CAD build for the part. Positions are in the model's coordinates, mm. A direction names the side the tool comes from. Coordinates: 2 decimals unless noted, no trailing zeros. Order: outer loops, then holes, each group sorted by start corner. A loop starts at its lowest first (then second) coordinate and runs counter-clockwise, first axis right, second up. Notation, with made-up numbers: (83, 16) - (136, 16) arc R18 cw to (136, 23) - close; hole circle Ø6 at (47.25, -35.5). An arc over 180 degrees is marked (long way). Write each question's results on one line, items separated by ' | '. Start each with the question number.
Q1. Band-saw the part on A-A, the plane x = 38.1. Write the cut outline in (y, z), then the cut area to 3 significant figures.
Q2. Band-saw the part on B-B, the plane x = 22. Write the cut outline in (y, z), then the cut area to 3 significant figures.
Q3. Band-saw the part on C-C, the plane x = 47. Write the cut outline in (y, z).
Q4. Wall check: probe 1 along Y at (x, z) = (12.7, 0.85); probe 2 along Z at (x, y) = (30, 9.25); probe 3 along Y at (x, z) = (31, 2.2). Give the ranges that are in metal, low to high.
Q5. Which spindle directions (+Z, -Z, +X, -X, +Y, -Y) get a long thin tool onto all of the face, cutting with end or side? Do faces 5 (the flat face through (9.9, 8, 2)), 6 (the flat face through (47, 2, 2.6)), 7 (the flat face through (31.39, 8, 2)), 8 (the flat face through (47, 9.05, 2)). Say none if no direction does.
Q6. Pull direction X, two halves, no side cores. Call faces 1 (the flat face through (16, 4, 2.4)), 2 (the flat face through (0.9, 8, 2)), 3 (the flat face through (8, 7.55, 2)), 4 (the flat face through (29, 4, 2.4)): released by +X, released by -X, zero draft, split by the parting line, or undercut.
Q7. Pin check, flat tips, straight feed: P1, Ø3, axis at x = 22.225, y = 3.81, coming from the +Z side; P2, Ø0.5, axis at x = 9, z = 2, coming from the -Y side; P3, Ø0.8, axis at y = 8, z = 2.5, coming from the +X side. Stop position of each tip, or through.
Autodesk Fusion 360 part; units mm, degrees
sketch "Sketch1" plane through (0, 0, 0) normal (0, 0, 1) x (1, 0, 0)
  line L0 (0, 0) -> (50.8, 0)
  line L1 (50.8, 0) -> (50.8, 10.16)
  line L2 (50.8, 10.16) -> (0, 10.16)
  line L3 (0, 10.16) -> (0, 0)
  line L4 (25.4, 10.16) -> (25.4, 0) construction
  circle A0 centre (12.7, 8.128) radius 1.1
  circle A1 centre (38.1, 8.128) radius 1.1
  dimension "d1" = 50.8
  dimension "d2" = 10.16
  dimension "d3" = 2.2
  dimension "d4" = 2.2
  dimension "d5" = 12.7
  dimension "d6" = 38.1
  dimension "d7" = 8.128
  dimension "d8" = 8.128
extrude "Extrude1" add sketch "Sketch1" along normal blind 1.6
sketch "Sketch2" plane through (0, 0, 1.6) normal (0, 0, 1) x (-1, 0, 0)
  circle A0 centre (-12.7, -8.128) radius 1.1
  circle A1 centre (-38.1, -8.128) radius 1.1
  line L0 (0, -10.16) -> (0, 0)
  line L1 (0, 0) -> (-50.8, 0)
  line L2 (-50.8, 0) -> (-50.8, -10.16)
  line L3 (-50.8, -10.16) -> (0, -10.16)
  line L4 (-5.675, -1.31) -> (-0.675, -1.31)
  line L5 (-0.675, -1.31) -> (-0.675, -6.31)
  line L6 (-0.675, -6.31) -> (-5.675, -6.31)
  line L7 (-5.675, -6.31) -> (-5.675, -1.31)
  line L8 (-5.675, -1.31) -> (-0.675, -6.31) construction
  line L9 (-0.675, -1.31) -> (-5.675, -6.31) construction
  circle A2 centre (-3.175, -3.81) radius 1.75
  line L10 (-7.025, -1.31) -> (-7.025, -6.31)
  line L11 (-7.025, -6.31) -> (-12.025, -6.31)
  line L12 (-12.025, -1.31) -> (-7.025, -1.31)
  line L13 (-12.025, -6.31) -> (-12.025, -1.31)
  circle A3 centre (-9.525, -3.81) radius 1.75
  line L14 (-13.375, -1.31) -> (-13.375, -6.31)
  line L15 (-13.375, -6.31) -> (-18.375, -6.31)
  line L16 (-18.375, -1.31) -> (-13.375, -1.31)
  line L17 (-18.375, -6.31) -> (-18.375, -1.31)
  circle A4 centre (-15.875, -3.81) radius 1.75
  line L18 (-19.725, -1.31) -> (-19.725, -6.31)
  line L19 (-19.725, -6.31) -> (-24.725, -6.31)
  line L20 (-24.725, -1.31) -> (-19.725, -1.31)
  line L21 (-24.725, -6.31) -> (-24.725, -1.31)
  circle A5 centre (-22.225, -3.81) radius 1.75
  line L22 (-26.075, -1.31) -> (-26.075, -6.31)
  line L23 (-26.075, -6.31) -> (-31.075, -6.31)
  line L24 (-31.075, -1.31) -> (-26.075, -1.31)
  line L25 (-31.075, -6.31) -> (-31.075, -1.31)
  circle A6 centre (-28.575, -3.81) radius 1.75
  line L26 (-32.425, -1.31) -> (-32.425, -6.31)
  line L27 (-32.425, -6.31) -> (-37.425, -6.31)
  line L28 (-37.425, -1.31) -> (-32.425, -1.31)
  line L29 (-37.425, -6.31) -> (-37.425, -1.31)
  circle A7 centre (-34.925, -3.81) radius 1.75
  line L30 (-38.775, -1.31) -> (-38.775, -6.31)
  line L31 (-38.775, -6.31) -> (-43.775, -6.31)
  line L32 (-43.775, -1.31) -> (-38.775, -1.31)
  line L33 (-43.775, -6.31) -> (-43.775, -1.31)
  circle A8 centre (-41.275, -3.81) radius 1.75
  line L34 (-45.125, -1.31) -> (-45.125, -6.31)
  line L35 (-45.125, -6.31) -> (-50.125, -6.31)
  line L36 (-50.125, -1.31) -> (-45.125, -1.31)
  line L37 (-50.125, -6.31) -> (-50.125, -1.31)
  circle A9 centre (-47.625, -3.81) radius 1.75
  point P0 (-3.175, -3.81)
  dimension "d13" = 5
  dimension "d14" = 5
  dimension "d15" = 3.175
  dimension "d16" = 3.81
  dimension "d17" = 3.5
  dimension "d20" = -6.35
  dimension "d21" = 0
extrude "Extrude2" add sketch "Sketch2" along normal blind 1 draft 1 contours L4 L5 L6 L7 | A2 | L10 L11 L12 L13 | A3 | L14 L15 L16 L17 | A4 | L18 L19 L20 L21 | A5 | L22 L23 L24 L25 | A6 | L26 L27 L28 L29 | A7 | L30 L31 L32 L33 | A8 | L34 L35 L36 L37 | A9
extrude "Extrude3" cut sketch "Sketch2" against normal blind 0.2 from surface at 1 contours A2 | A3 | A4 | A5 | A6 | A7 | A8 | A9
sketch "Sketch3" plane through (0, 0, 1.6) normal (0, 0, 1) x (-1, 0, 0)
  line L0 (-50.125, -6.31) -> (-50.125, -1.31)
  line L1 (-50.125, -1.31) -> (-45.125, -1.31)
  line L2 (-45.125, -1.31) -> (-45.125, -6.31)
  line L3 (-45.125, -6.31) -> (-50.125, -6.31)
  line L4 (-24.725, -6.31) -> (-24.725, -1.31)
  line L5 (-24.725, -1.31) -> (-19.725, -1.31)
  line L6 (-19.725, -1.31) -> (-19.725, -6.31)
  line L7 (-19.725, -6.31) -> (-24.725, -6.31)
  line L8 (-5.675, -6.31) -> (-5.675, -1.31)
  line L9 (-5.675, -1.31) -> (-0.675, -1.31)
  line L10 (-0.675, -1.31) -> (-0.675, -6.31)
  line L11 (-0.675, -6.31) -> (-5.675, -6.31)
  line L12 (-31.075, -6.31) -> (-31.075, -1.31)
  line L13 (-31.075, -1.31) -> (-26.075, -1.31)
  line L14 (-26.075, -1.31) -> (-26.075, -6.31)
  line L15 (-26.075, -6.31) -> (-31.075, -6.31)
  line L16 (-43.775, -6.31) -> (-43.775, -1.31)
  line L17 (-43.775, -1.31) -> (-38.775, -1.31)
  line L18 (-38.775, -1.31) -> (-38.775, -6.31)
  line L19 (-38.775, -6.31) -> (-43.775, -6.31)
  line L20 (-18.375, -6.31) -> (-18.375, -1.31)
  line L21 (-18.375, -1.31) -> (-13.375, -1.31)
  line L22 (-13.375, -1.31) -> (-13.375, -6.31)
  line L23 (-13.375, -6.31) -> (-18.375, -6.31)
  line L24 (-12.025, -6.31) -> (-12.025, -1.31)
  line L25 (-12.025, -1.31) -> (-7.025, -1.31)
  line L26 (-7.025, -1.31) -> (-7.025, -6.31)
  line L27 (-7.025, -6.31) -> (-12.025, -6.31)
  line L28 (-37.425, -6.31) -> (-37.425, -1.31)
  line L29 (-37.425, -1.31) -> (-32.425, -1.31)
  line L30 (-32.425, -1.31) -> (-32.425, -6.31)
  line L31 (-32.425, -6.31) -> (-37.425, -6.31)
  circle A0 centre (-12.7, -8.128) radius 1.1
  circle A1 centre (-38.1, -8.128) radius 1.1
  line L32 (0, -10.16) -> (0, 0)
  line L33 (0, 0) -> (-50.8, 0)
  line L34 (-50.8, 0) -> (-50.8, -10.16)
  line L35 (-50.8, -10.16) -> (0, -10.16)
  line L36 (-0.9, -9.05) -> (-3.9, -9.05)
  line L37 (-3.9, -9.05) -> (-3.9, -7.55)
  line L38 (-3.9, -7.55) -> (-0.9, -7.55)
  line L39 (-0.9, -7.55) -> (-0.9, -9.05)
  line L40 (-2.4, -9.05) -> (-2.4, -7.55) construction
  line L41 (-3.9, -8.3) -> (-0.9, -8.3) construction
  line L42 (-6.9, -7.55) -> (-6.9, -9.05)
  line L43 (-6.9, -9.05) -> (-9.9, -9.05)
  line L44 (-9.9, -7.55) -> (-6.9, -7.55)
  line L45 (-9.9, -9.05) -> (-9.9, -7.55)
  line L46 (-15.4, -9.05) -> (-18.4, -9.05)
  line L47 (-18.4, -9.05) -> (-18.4, -7.55)
  line L48 (-18.4, -7.55) -> (-15.4, -7.55)
  line L49 (-15.4, -7.55) -> (-15.4, -9.05)
  line L50 (-16.9, -9.05) -> (-16.9, -7.55) construction
  line L51 (-18.4, -8.3) -> (-15.4, -8.3) construction
  line L52 (-23.73, -7.55) -> (-20.73, -7.55)
  line L53 (-20.73, -7.55) -> (-20.73, -9.05)
  line L54 (-20.73, -9.05) -> (-23.73, -9.05)
  line L55 (-23.73, -9.05) -> (-23.73, -7.55)
  line L56 (-29.06, -7.55) -> (-26.06, -7.55)
  line L57 (-26.06, -7.55) -> (-26.06, -9.05)
  line L58 (-26.06, -9.05) -> (-29.06, -9.05)
  line L59 (-29.06, -9.05) -> (-29.06, -7.55)
  line L60 (-34.39, -7.55) -> (-31.39, -7.55)
  line L61 (-31.39, -7.55) -> (-31.39, -9.05)
  line L62 (-31.39, -9.05) -> (-34.39, -9.05)
  line L63 (-34.39, -9.05) -> (-34.39, -7.55)
  line L64 (-39.72, -9.05) -> (-42.72, -9.05)
  line L65 (-42.72, -9.05) -> (-42.72, -7.55)
  line L66 (-42.72, -7.55) -> (-39.72, -7.55)
  line L67 (-39.72, -7.55) -> (-39.72, -9.05)
  line L68 (-41.22, -9.05) -> (-41.22, -7.55) construction
  line L69 (-39.72, -8.3) -> (-42.72, -8.3) construction
  line L70 (-32.89, -9.05) -> (-32.89, -7.55) construction
  line L71 (-45.94, -7.55) -> (-45.94, -9.05)
  line L72 (-45.94, -9.05) -> (-48.94, -9.05)
  line L73 (-48.94, -7.55) -> (-45.94, -7.55)
  line L74 (-48.94, -9.05) -> (-48.94, -7.55)
  dimension "d27" = 3
  dimension "d28" = 1.5
  dimension "d29" = 2.4
  dimension "d30" = 8.3
  dimension "d33" = -6
  dimension "d34" = 0
  dimension "d35" = 3
  dimension "d36" = 1.5
  dimension "d37" = 14.5
  dimension "d40" = -5.33
  dimension "d41" = 0
  dimension "d42" = 3
  dimension "d43" = 1.5
  dimension "d44" = 8.33
  dimension "d47" = -6.22
  dimension "d48" = 0
extrude "Extrude4" add sketch "Sketch3" along normal blind 1 contours L36 L37 L38 L39 | L42 L43 L44 L45 | L46 L47 L48 L49 | L52 L53 L54 L55 | L56 L57 L58 L59 | L60 L61 L62 L63 | L64 L65 L66 L67 | L71 L72 L73 L74
Results below:
1) outline: (0, 0) - (7.03, 0) - (7.03, 1.6) - (0, 1.6) - close; (9.23, 0) - (10.16, 0) - (10.16, 1.6) - (9.23, 1.6) - close | area: 12.7 mm²
2) outline: (0, 0) - (10.16, 0) - (10.16, 1.6) - (9.05, 1.6) - (9.05, 2.6) - (7.55, 2.6) - (7.55, 1.6) - (6.31, 1.6) - (6.33, 2.6) - (5.55, 2.6) - (5.55, 2.4) - (2.07, 2.4) - (2.07, 2.6) - (1.29, 2.6) - (1.31, 1.6) - (0, 1.6) - close | area: 22.1 mm²
3) outline: (0, 0) - (10.16, 0) - (10.16, 1.6) - (9.05, 1.6) - (9.05, 2.6) - (7.55, 2.6) - (7.55, 1.6) - (6.31, 1.6) - (6.33, 2.6) - (5.44, 2.6) - (5.44, 2.4) - (2.18, 2.4) - (2.18, 2.6) - (1.29, 2.6) - (1.31, 1.6) - (0, 1.6) - close
4) probe 1: y = 0 to 7.03, 9.23 to 10.16 | probe 2: z = 0 to 1.6 | probe 3: y = 1.3 to 6.32
5) face 5: +Z, +Y | face 6: +Z, +X, -X, +Y, -Y | face 7: +Z, +Y, -Y | face 8: +Z, +X, -X, +Y
6) face 1: undercut | face 2: released by -X | face 3: zero draft | face 4: undercut
7) P1: stops at z = 2.4 | P2: stops at y = 1.3 | P3: stops at x = 48.94
